Design review of the part built by this model. Coordinates are the model's own, in mm. A direction names the side the tool comes from. Coordinates: 2 decimals unless noted, no trailing zeros. Order: outer loops, then holes, each group sorted by start corner. A loop starts at its lowest first (then second) coordinate and runs counter-clockwise, first axis right, second up. Notation, with made-up numbers: (-16, -12) -> (14, -12) arc R27 cw to (14, 20) -> close; hole circle Ø4 at (-37, 40). An arc over 180 degrees is marked (long way). Use a Markdown table: item, result. Add a question column.
Q1. Add section C-C (z = 1.6). State the section outline as (x, y) points.
Q2. Wall thickness on probe 1 along Y at (x, z) = (10, 2.5); probe 2 along Y at (x, z) = (107.95, 2.6); probe 3 along Y at (x, z) = (23, 2.1): over which ranges is each line inside the solid? List them lowest first.
Q3. Add section B-B (x = 48.26). State the section outline as (y, z) points.
Q4. Add section A-A (y = -57.15). State the section outline as (x, z) points.
Q5. Machinability: for faces 5 (the face through (58, 12.7, 2)), 6 (the face through (7.57, 4.364, 2.348)), 7 (the face through (114.3, -58, 2)), 8 (the face through (101.6, -25, 2)), which of the approach directions +Z, -Z, +X, -X, +Y, -Y give a long, thin tool a straight path to every point of the face, cutting with its end or side? Answer none if there is none.
Q6. Insertion check: pin 1 (4 mm diameter, centred on x = 107.95, y = -6.35, fed in from +Z); pin 2 (1.4 mm diameter, centred on y = -60, z = 1.5, fed in from +X); pin 3 (2.5 mm diameter, centred on x = 85, z = 3, fed in from +Y). Each pin has a flat end and moves straight along its axis. Give the tip position at first contact, or say it passes through.
Q7. The part is to be moulded in two halves that separate along X. For faces 1 (the face through (168.53, 15.25, 2.35)), 2 (the face through (50, 0, 2)), 3 (the face through (47.835, -53.914, 2.348)), 4 (the face through (133.99, 25.76, 2.35)), say which applies: pulls with the +X half, pulls with the -X half, needs draft (parallel to the pull), parting line crosses it, or undercut.
Q8. Add section D-D (x = 83). State the section outline as (y, z) points, then the cut area to 3 significant figures.
from build123d import *

# Parameters (mm, degrees)
SKETCH1_R           = 3.2639
BOSS_EXTRUDE1_DEPTH = 4.7625
CUT_EXTRUDE1_REACH  = 6.763
SKETCH2_R           = 3.2639


with BuildPart() as part:
    # Sketch1 → Boss-Extrude1 (new body)
    with BuildSketch(Plane.XY):
        Polygon((0, 0), (101.6, 0), (101.6, -50.8), (0, -50.8), (0, -63.5), (114.3, -63.5), (114.3, -53.215281422), (183.499345052, -7.322414016), (153.138236671, 38.457440977), (114.3, 12.7), (0, 12.7), align=None)
        with Locations((10.16, 6.35)):
            Circle(SKETCH1_R, mode=Mode.SUBTRACT)
        with Locations((48.26, 6.35)):
            Circle(SKETCH1_R, mode=Mode.SUBTRACT)
        with Locations((10.16, -57.15)):
            Circle(SKETCH1_R, mode=Mode.SUBTRACT)
        with Locations((48.26, -57.15)):
            Circle(SKETCH1_R, mode=Mode.SUBTRACT)
    extrude(amount=BOSS_EXTRUDE1_DEPTH)

    # Sketch2 → Cut-Extrude1 (cut, up to next)
    with BuildSketch(Plane.XY.offset(4.7625), mode=Mode.PRIVATE) as cut_extrude1_sk1:
        with Locations((107.95, -6.35)):
            Circle(SKETCH2_R)
    cut_extrude1_tool1 = extrude(cut_extrude1_sk1.sketch, amount=-CUT_EXTRUDE1_REACH, mode=Mode.PRIVATE) & part.part
    add(cut_extrude1_tool1.solids().sort_by_distance((107.95, -6.35, 4.7625))[0], mode=Mode.SUBTRACT)
    # Sketch2 → Cut-Extrude1 (cut, up to next)
    with BuildSketch(Plane.XY.offset(4.7625), mode=Mode.PRIVATE) as cut_extrude1_sk2:
        with Locations((107.95, -44.45)):
            Circle(SKETCH2_R)
    cut_extrude1_tool2 = extrude(cut_extrude1_sk2.sketch, amount=-CUT_EXTRUDE1_REACH, mode=Mode.PRIVATE) & part.part
    add(cut_extrude1_tool2.solids().sort_by_distance((107.95, -44.45, 4.7625))[0], mode=Mode.SUBTRACT)


solid = part.part
Established:
| question | item | result |
|---|---|---|
| 1 | outline | (0, -63.5) -> (114.3, -63.5) -> (114.3, -53.22) -> (183.5, -7.32) -> (153.14, 38.46) -> (114.3, 12.7) -> (0, 12.7) -> (0, 0) -> (101.6, 0) -> (101.6, -50.8) -> (0, -50.8) -> close; hole circle Ø6.53 at (10.16, -57.15); hole circle Ø6.53 at (10.16, 6.35); hole circle Ø6.53 at (48.26, -57.15); hole circle Ø6.53 at (48.26, 6.35); hole circle Ø6.53 at (107.95, -44.45); hole circle Ø6.53 at (107.95, -6.35) |
| 2 | probe 1 | -63.5 to -60.41, -53.89 to -50.8, 0 to 3.09, 9.61 to 12.7 |
| 2 | probe 2 | -63.5 to -47.71, -41.19 to -9.61, -3.09 to 12.7 |
| 2 | probe 3 | -63.5 to -50.8, 0 to 12.7 |
| 3 | outline | (-63.5, 0) -> (-60.41, 0) -> (-60.41, 4.76) -> (-63.5, 4.76) -> close; (-53.89, 0) -> (-50.8, 0) -> (-50.8, 4.76) -> (-53.89, 4.76) -> close; (0, 0) -> (3.09, 0) -> (3.09, 4.76) -> (0, 4.76) -> close; (9.61, 0) -> (12.7, 0) -> (12.7, 4.76) -> (9.61, 4.76) -> close |
| 4 | outline | (0, 0) -> (6.9, 0) -> (6.9, 4.76) -> (0, 4.76) -> close; (13.42, 0) -> (45, 0) -> (45, 4.76) -> (13.42, 4.76) -> close; (51.52, 0) -> (114.3, 0) -> (114.3, 4.76) -> (51.52, 4.76) -> close |
| 5 | face 5 | +Z, -Z, -X, +Y |
| 5 | face 6 | +Z, -Z |
| 5 | face 7 | +Z, -Z, +X, -Y |
| 5 | face 8 | +Z, -Z, -X |
| 6 | pin 1 | through |
| 6 | pin 2 | x = 114.3 |
| 6 | pin 3 | y = 12.7 |
| 7 | face 1 | pulls with the +X half |
| 7 | face 2 | needs draft |
| 7 | face 3 | undercut |
| 7 | face 4 | pulls with the -X half |
| 8 | outline | (-63.5, 0) -> (-50.8, 0) -> (-50.8, 4.76) -> (-63.5, 4.76) -> close; (0, 0) -> (12.7, 0) -> (12.7, 4.76) -> (0, 4.76) -> close |
| 8 | area | 121 mm^2 |
